Part model, mm, in its own coordinate system. A direction names the side the tool comes from. Give positions to 0.01 mm unless a question says otherwise; leave off trailing zeros. Loops run counter-clockwise (first coordinate to the right, second up) from the corner with the lowest first, then second, coordinate; pieces in that order, holes last. Notation, with made-up numbers: (27.25, -3.5) -> (32.25, -3.5) arc R6 cw to (32.25, 3.5) -> close; hole circle Ø3 at (-7.5, -11). An arc over 180 degrees is marked (long way). One line per question, with ' | ' between items.
```python
from build123d import *

# Parameters (mm, degrees)
SKETCH1_W            = 37.9349
SKETCH1_H            = 37.9349
BOSS_EXTRUDE1_DEPTH  = 1.651
SKETCH2_W            = 16.002
SKETCH2_H            = 16.002
BOSS_EXTRUDE2_DEPTH  = 7.62
SKETCH3_R            = 8.001
BOSS_EXTRUDE3_DEPTH  = 6.35
SKETCH4_R            = 5.9309
BOSS_EXTRUDE4_DEPTH  = 4.9403
SKETCH5_R            = 6.985
BOSS_EXTRUDE5_DEPTH  = 4.2545
SKETCH6_R            = 4.38785
CUT_EXTRUDE1_DEPTH   = 0.635
FILLET2_R            = 2.54
SKETCH9_R            = 1.1176
CUT_EXTRUDE2_DEPTH   = 1.651
SKETCH12_W           = 3.3274
SKETCH12_H           = 4.5466
BOSS_EXTRUDE6_DEPTH  = 3.6957
SKETCH13_W           = 10.16
SKETCH13_H           = 4.7117
BOSS_EXTRUDE7_DEPTH  = 5.6515
SKETCH14_W           = 4.8006
SKETCH14_H           = 6.0833
BOSS_EXTRUDE8_DEPTH  = 5.842
SKETCH15_W           = 3.3528
SKETCH15_H           = 4.5212
BOSS_EXTRUDE9_DEPTH  = 4.6101
BOSS_EXTRUDE10_DEPTH = 4.1402


# Read off the part's stored shape, not the designer's step: Dome1
with BuildPart() as part:
    # Sketch1 → Boss-Extrude1 (new body)
    with BuildSketch(Plane.XY):
        with Locations((18.96745, 18.96745)):
            Rectangle(SKETCH1_W, SKETCH1_H)
    extrude(amount=BOSS_EXTRUDE1_DEPTH)

    # Sketch2 → Boss-Extrude2 (add)
    with BuildSketch(Plane.XY.offset(1.651)):
        with Locations((18.96745, 18.96745)):
            Rectangle(SKETCH2_W, SKETCH2_H)
    extrude(amount=BOSS_EXTRUDE2_DEPTH)

    # Sketch3 → Boss-Extrude3 (add)
    with BuildSketch(Plane.XY.offset(9.271)):
        with Locations((18.96745, 18.96745)):
            Circle(SKETCH3_R)
    extrude(amount=BOSS_EXTRUDE3_DEPTH)

    # Sketch4 → Boss-Extrude4 (add)
    with BuildSketch(Plane.XY.offset(15.621)):
        with Locations((18.96745, 18.96745)):
            Circle(SKETCH4_R)
    extrude(amount=BOSS_EXTRUDE4_DEPTH)

    # Sketch5 → Boss-Extrude5 (add)
    with BuildSketch(Plane.XY.offset(20.5613)):
        with Locations((18.96745, 18.96745)):
            Circle(SKETCH5_R)
    extrude(amount=BOSS_EXTRUDE5_DEPTH)

    # Sketch6 → Cut-Extrude1 (cut)
    with BuildSketch(Plane.XY.offset(24.8158)):
        with Locations((18.96745, 18.96745)):
            Circle(SKETCH6_R)
    extrude(amount=-CUT_EXTRUDE1_DEPTH, mode=Mode.SUBTRACT)

    # Fillet2
    # the kernel refuses this fillet: 2.54 mm, written as the material it takes off along each edge
    with BuildSketch(Plane(origin=(18.96745, 18.96745, 24.8158), x_dir=(1, 0, 0), z_dir=(0, -1, 0))) as fillet2_piece_1:
        with BuildLine():
            CenterArc((6.067902083, -2.54), FILLET2_R, 90, 41.409622109)
            Line((4.38785, -0.635), (4.354248958, -0.5969))
            ThreePointArc((4.354248958, -0.5969), (4.33705, -0.3175), (4.33705, 0))
            Line((4.33705, 0), (4.38785, 0.0508))
            Line((4.38785, 0.0508), (6.067902083, 0.0508))
            Line((6.067902083, 0.0508), (6.067902083, 0))
        make_face()
    revolve(axis=Axis((18.96745, 18.96745, 24.8158), (0, 0, 1)), mode=Mode.SUBTRACT)

    # Dome1 outline → Dome1 (revolve)
    with BuildSketch(Plane(origin=(18.96745, 18.96745, 0), x_dir=(1, 0, 0), z_dir=(0, -1, 0))):
        with BuildLine():
            Line((0, 24.1808), (4.387850012, 24.180799996))
            ThreePointArc((4.387850012, 24.180799996), (2.22676176, 24.75088497), (0, 24.9428))
            Line((0, 24.9428), (0, 24.1808))
        make_face()
    revolve(axis=Axis((18.96745, 18.96745, 0), (0, 0, 1)))

    # Sketch9 → Cut-Extrude2 (cut)
    with BuildSketch(Plane.XY.offset(1.651)):
        with Locations((33.62325, 33.62325)):
            Circle(SKETCH9_R)
        with Locations((4.31165, 33.62325)):
            Circle(SKETCH9_R)
        with Locations((4.31165, 4.31165)):
            Circle(SKETCH9_R)
        with Locations((33.62325, 4.31165)):
            Circle(SKETCH9_R)
        with BuildLine():
            Line((35.385619933, 12.100169933), (35.385619933, 2.549280067))
            Line((35.385619933, 2.549280067), (25.834730067, 2.549280067))
            ThreePointArc((25.834730067, 2.549280067), (25.2984, 2.01295), (25.834730067, 1.476619933))
            Line((25.834730067, 1.476619933), (35.385619933, 1.476619933))
            ThreePointArc((35.385619933, 1.476619933), (37.303202335, 0.631697665), (36.458280067, 2.549280067))
            Line((36.458280067, 2.549280067), (36.458280067, 12.100169933))
            ThreePointArc((36.458280067, 12.100169933), (35.92195, 12.6365), (35.385619933, 12.100169933))
        make_face()
        with BuildLine():
            Line((35.385619933, 36.458280067), (25.834730067, 36.458280067))
            ThreePointArc((25.834730067, 36.458280067), (25.2984, 35.92195), (25.834730067, 35.385619933))
            Line((25.834730067, 35.385619933), (35.385619933, 35.385619933))
            Line((35.385619933, 35.385619933), (35.385619933, 25.834730067))
            ThreePointArc((35.385619933, 25.834730067), (35.92195, 25.2984), (36.458280067, 25.834730067))
            Line((36.458280067, 25.834730067), (36.458280067, 35.385619933))
            ThreePointArc((36.458280067, 35.385619933), (37.303202335, 37.303202335), (35.385619933, 36.458280067))
        make_face()
        with BuildLine():
            Line((12.048880067, 36.458280067), (2.549280067, 36.458280067))
            ThreePointArc((2.549280067, 36.458280067), (0.631697665, 37.303202335), (1.476619933, 35.385619933))
            Line((1.476619933, 35.385619933), (1.476619933, 25.886019933))
            ThreePointArc((1.476619933, 25.886019933), (2.01295, 25.349689867), (2.549280067, 25.886019933))
            Line((2.549280067, 25.886019933), (2.549280067, 35.385619933))
            Line((2.549280067, 35.385619933), (12.048880067, 35.385619933))
            ThreePointArc((12.048880067, 35.385619933), (12.585210133, 35.92195), (12.048880067, 36.458280067))
        make_face()
        with BuildLine():
            Line((23.06955, 36.458280067), (14.86535, 36.458280067))
            ThreePointArc((14.86535, 36.458280067), (14.329019933, 35.92195), (14.86535, 35.385619933))
            Line((14.86535, 35.385619933), (23.06955, 35.385619933))
            ThreePointArc((23.06955, 35.385619933), (23.605880067, 35.92195), (23.06955, 36.458280067))
        make_face()
        with BuildLine():
            Line((2.549280067, 23.06955), (2.549280067, 14.86535))
            ThreePointArc((2.549280067, 14.86535), (2.01295, 14.329019933), (1.476619933, 14.86535))
            Line((1.476619933, 14.86535), (1.476619933, 23.06955))
            ThreePointArc((1.476619933, 23.06955), (2.01295, 23.605880067), (2.549280067, 23.06955))
        make_face()
        with BuildLine():
            Line((36.458280067, 23.06955), (36.458280067, 14.86535))
            ThreePointArc((36.458280067, 14.86535), (35.92195, 14.329019933), (35.385619933, 14.86535))
            Line((35.385619933, 14.86535), (35.385619933, 23.06955))
            ThreePointArc((35.385619933, 23.06955), (35.92195, 23.605880067), (36.458280067, 23.06955))
        make_face()
        with BuildLine():
            Line((23.06955, 2.549280067), (14.86535, 2.549280067))
            ThreePointArc((14.86535, 2.549280067), (14.329019933, 2.01295), (14.86535, 1.476619933))
            Line((14.86535, 1.476619933), (23.06955, 1.476619933))
            ThreePointArc((23.06955, 1.476619933), (23.605880067, 2.01295), (23.06955, 2.549280067))
        make_face()
        with BuildLine():
            Line((2.549280067, 12.100169933), (2.549280067, 2.549280067))
            Line((2.549280067, 2.549280067), (12.100169933, 2.549280067))
            ThreePointArc((12.100169933, 2.549280067), (12.6365, 2.01295), (12.100169933, 1.476619933))
            Line((12.100169933, 1.476619933), (2.600569933, 1.476619933))
            ThreePointArc((2.600569933, 1.476619933), (0.681867267, 0.681867267), (1.476619933, 2.600569933))
            Line((1.476619933, 2.600569933), (1.476619933, 12.100169933))
            ThreePointArc((1.476619933, 12.100169933), (2.01295, 12.6365), (2.549280067, 12.100169933))
        make_face()
    extrude(amount=-CUT_EXTRUDE2_DEPTH, mode=Mode.SUBTRACT)

    # Sketch12 → Boss-Extrude6 (add)
    with BuildSketch(Plane(origin=(0, 0, 0), x_dir=(-1, 0, 0), z_dir=(0, 0, -1))):
        with Locations((-33.721919933, 18.96745)):
            Rectangle(SKETCH12_W, SKETCH12_H)
    extrude(amount=BOSS_EXTRUDE6_DEPTH)

    # Sketch13 → Boss-Extrude7 (add)
    with BuildSketch(Plane(origin=(0, 0, 0), x_dir=(-1, 0, 0), z_dir=(0, 0, -1))):
        with Locations((-23.8125, 4.905130067)):
            Rectangle(SKETCH13_W, SKETCH13_H)
    extrude(amount=BOSS_EXTRUDE7_DEPTH)

    # Sketch14 → Boss-Extrude8 (add)
    with BuildSketch(Plane(origin=(0, 0, 0), x_dir=(-1, 0, 0), z_dir=(0, 0, -1))):
        with Locations((-4.949580067, 12.02055)):
            Rectangle(SKETCH14_W, SKETCH14_H)
    extrude(amount=BOSS_EXTRUDE8_DEPTH)

    # Sketch15 → Boss-Extrude9 (add)
    with BuildSketch(Plane(origin=(0, 0, 0), x_dir=(-1, 0, 0), z_dir=(0, 0, -1))):
        with Locations((-4.225680067, 17.3228)):
            Rectangle(SKETCH15_W, SKETCH15_H)
    extrude(amount=BOSS_EXTRUDE9_DEPTH)

    # Sketch16 → Boss-Extrude10 (add)
    with BuildSketch(Plane.XY.offset(1.651)):
        with BuildLine():
            Line((26.96845, 16.9545), (28.30703, 16.9545))
            ThreePointArc((28.30703, 16.9545), (30.31998, 18.96745), (28.30703, 20.9804))
            Line((28.30703, 20.9804), (26.96845, 20.9804))
            Line((26.96845, 20.9804), (26.96845, 16.9545))
        make_face()
        with BuildLine():
            Line((9.62787, 20.9804), (10.96645, 20.9804))
            Line((10.96645, 20.9804), (10.96645, 16.9545))
            Line((10.96645, 16.9545), (9.62787, 16.9545))
            ThreePointArc((9.62787, 16.9545), (7.61492, 18.96745), (9.62787, 20.9804))
        make_face()
    extrude(amount=BOSS_EXTRUDE10_DEPTH)


solid = part.part
```
1) Pin check, flat tips, straight feed: P1, Ø3, axis at x = 8.5, z = 15, coming from the +Y side; P2, Ø12, axis at x = 18, y = 16, coming from the -Z side; P3, Ø1, axis at y = 16.5, z = 14, coming from the -X side; P4, Ø2, axis at x = 14, y = 18, coming from the +Z side. Stop position of each tip, or through.
Found:
P1: through | P2: z = 0 | P3: x = 11.21 | P4: z = 24.82
2) Tool access for faces 1 (the cylindrical face through (13.42, 14.72, 22.66)), 2 (the flat face through (10, 16.954, 4)), 3 (the cylindrical face through (2, 25.35, 0.84)): list every direction of +Z, -Z, +X, -X, +Y, -Y with a clear straight run to the whole face (end or side of a thin tool).
Found:
face 1: +Z | face 2: +Z, -X, -Y | face 3: +Z, -Z
3) Saw through at D-D (z = 18). Give the cut face in (x, y).
Found:
outline: circle Ø11.86 at (18.97, 18.97)
4) Saw through at C-C (z = 3.5). Give the cut face in (x, y).
Found:
outline: (9.63, 16.95) -> (10.97, 16.95) -> (10.97, 10.97) -> (26.97, 10.97) -> (26.97, 16.95) -> (28.31, 16.95) arc R2.01 ccw to (28.31, 20.98) -> (26.97, 20.98) -> (26.97, 26.97) -> (10.97, 26.97) -> (10.97, 20.98) -> (9.63, 20.98) arc R2.01 ccw to start
5) Pull direction X, two halves, no side cores. Call faces 4 (the flat face through (37.935, 19, 1)), 5 (the flat face through (1.477, 31, 1)), 6 (the flat face through (7, 36.458, 1)), 7 (the flat face through (25, 25, 9.271)): pulls with the +X half, pulls with the -X half, needs draft (parallel to the pull), parting line crosses it, or undercut.
Found:
face 4: pulls with the +X half | face 5: undercut | face 6: undercut | face 7: needs draft
6) Saw through at B-B (y = 29). Give the cut face in (x, z), and give its area (3 significant figures).
Found:
outline: (0, 0) -> (1.48, 0) -> (1.48, 1.65) -> (0, 1.65) -> close; (2.55, 0) -> (35.39, 0) -> (35.39, 1.65) -> (2.55, 1.65) -> close; (36.46, 0) -> (37.93, 0) -> (37.93, 1.65) -> (36.46, 1.65) -> close | area: 59.1 mm2
7) Saw through at A-A (x = 27.5). Give the cut face in (y, z), and give its area (3 significant figures).
Found:
outline: (0, 0) -> (1.48, 0) -> (1.48, 1.65) -> (0, 1.65) -> close; (2.55, -5.65) -> (7.26, -5.65) -> (7.26, 0) -> (35.39, 0) -> (35.39, 1.65) -> (20.98, 1.65) -> (20.98, 5.79) -> (16.95, 5.79) -> (16.95, 1.65) -> (2.55, 1.65) -> close; (36.46, 0) -> (37.93, 0) -> (37.93, 1.65) -> (36.46, 1.65) -> close | area: 102 mm2
8) Drill centre lines: line 1 (Z direction, x = 19.5, y = 25.5); line 2 (Z direction, x = 15, y = 9.5); line 3 (X direction, y = 18.5, z = -0.5). Where is each one in solid material? Low to high.
Found:
line 1: 0 to 15.62, 20.56 to 24.82 | line 2: 0 to 1.65 | line 3: 2.55 to 5.9, 32.06 to 35.39
